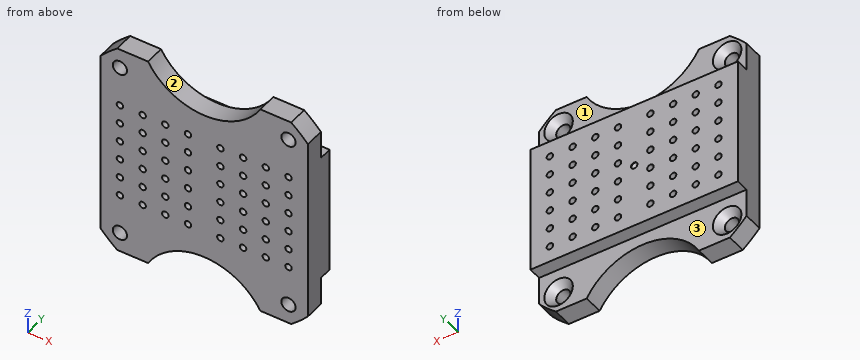
from build123d import *

# Parameters (mm, degrees)
SKIZZE1_W                                            = 32
SKIZZE1_H                                            = 33.6
AUFSATZ_LINEAR_AUSTRAGEN1_DEPTH                      = 5
SKIZZE9_R                                            = 0.5
SCHNITT_LINEAR_AUSTRAGEN1_DEPTH                      = 6
SKIZZE10_W                                           = 32
SKIZZE10_H                                           = 6.8
SCHNITT_LINEAR_AUSTRAGEN2_DEPTH                      = 2
FORMSENKUNG_F_R_M2_LINSENSENKSCHRAUBE_MI_D           = 2.2
FORMSENKUNG_F_R_M2_LINSENSENKSCHRAUBE_MI_DEPTH       = 4
FORMSENKUNG_F_R_M2_LINSENSENKSCHRAUBE_MI_CSINK_D     = 4.4
FORMSENKUNG_F_R_M2_LINSENSENKSCHRAUBE_MI_CSINK_ANGLE = 90
FORMSENKUNG_F_R_M2_LINSENSENKSCHRAUBE_MI_TIP         = 0.660946681
SKIZZE13_R                                           = 10
SCHNITT_LINEAR_AUSTRAGEN3_DEPTH                      = 24.393161394
SKIZZE14_R                                           = 31.5
SKIZZE14_R_2                                         = 21.5
SCHNITT_LINEAR_AUSTRAGEN_D_NN1_DEPTH                 = 10
F_1_0_1_DURCHMESSER_BOHRUNG1_D                       = 1
F_1_0_1_DURCHMESSER_BOHRUNG1_DEPTH                   = 0.1
F_1_0_1_DURCHMESSER_BOHRUNG1_TIP                     = 0.30043031


with BuildPart() as part:
    # Skizze1 → Aufsatz-Linear austragen1 (new body)
    with BuildSketch(Plane(origin=(0, 0, 0), x_dir=(1, 0, 0), z_dir=(0, 1, 0))):
        Rectangle(SKIZZE1_W, SKIZZE1_H)
    extrude(amount=AUFSATZ_LINEAR_AUSTRAGEN1_DEPTH)

    # Skizze9 → Schnitt-Linear austragen1 (cut)
    with BuildSketch(Plane(origin=(0, 5, 0), x_dir=(1, 0, 0), z_dir=(0, 1, 0))):
        with Locations(Location((-13, 7.5, 0), (0, 0, 270))):
            Circle(SKIZZE9_R)
        with Locations(Location((-9.5, 7.5, 0), (0, 0, 270))):
            Circle(SKIZZE9_R)
        with Locations(Location((-6, 7.5, 0), (0, 0, 270))):
            Circle(SKIZZE9_R)
        with Locations(Location((-2.5, 7.5, 0), (0, 0, 270))):
            Circle(SKIZZE9_R)
        with Locations(Location((-2.5, 4.5, 0), (0, 0, 270))):
            Circle(SKIZZE9_R)
        with Locations(Location((13, -7.5, 0), (0, 0, 270))):
            Circle(SKIZZE9_R)
        with Locations(Location((13, -4.5, 0), (0, 0, 270))):
            Circle(SKIZZE9_R)
        with Locations(Location((13, -1.5, 0), (0, 0, 270))):
            Circle(SKIZZE9_R)
        with Locations(Location((13, 1.5, 0), (0, 0, 270))):
            Circle(SKIZZE9_R)
        with Locations(Location((13, 4.5, 0), (0, 0, 270))):
            Circle(SKIZZE9_R)
        with Locations(Location((-2.5, 1.5, 0), (0, 0, 270))):
            Circle(SKIZZE9_R)
        with Locations(Location((-9.5, 4.5, 0), (0, 0, 270))):
            Circle(SKIZZE9_R)
        with Locations(Location((-6, 4.5, 0), (0, 0, 270))):
            Circle(SKIZZE9_R)
        with Locations(Location((-2.5, -1.5, 0), (0, 0, 270))):
            Circle(SKIZZE9_R)
        with Locations(Location((-2.5, -4.5, 0), (0, 0, 270))):
            Circle(SKIZZE9_R)
        with Locations(Location((-2.5, -7.5, 0), (0, 0, 270))):
            Circle(SKIZZE9_R)
        with Locations(Location((6, -7.5, 0), (0, 0, 270))):
            Circle(SKIZZE9_R)
        with Locations(Location((9.5, -7.5, 0), (0, 0, 270))):
            Circle(SKIZZE9_R)
        with Locations(Location((2.5, -7.5, 0), (0, 0, 270))):
            Circle(SKIZZE9_R)
        with Locations(Location((2.5, -4.5, 0), (0, 0, 270))):
            Circle(SKIZZE9_R)
        with Locations(Location((6, -4.5, 0), (0, 0, 270))):
            Circle(SKIZZE9_R)
        with Locations(Location((-9.5, 1.5, 0), (0, 0, 270))):
            Circle(SKIZZE9_R)
        with Locations(Location((-6, 1.5, 0), (0, 0, 270))):
            Circle(SKIZZE9_R)
        with Locations(Location((2.5, -1.5, 0), (0, 0, 270))):
            Circle(SKIZZE9_R)
        with Locations(Location((2.5, 1.5, 0), (0, 0, 270))):
            Circle(SKIZZE9_R)
        with Locations(Location((9.5, -4.5, 0), (0, 0, 270))):
            Circle(SKIZZE9_R)
        with Locations(Location((2.5, 4.5, 0), (0, 0, 270))):
            Circle(SKIZZE9_R)
        with Locations(Location((2.5, 7.5, 0), (0, 0, 270))):
            Circle(SKIZZE9_R)
        with Locations(Location((6, -1.5, 0), (0, 0, 270))):
            Circle(SKIZZE9_R)
        with Locations(Location((9.5, -1.5, 0), (0, 0, 270))):
            Circle(SKIZZE9_R)
        with Locations(Location((-9.5, -1.5, 0), (0, 0, 270))):
            Circle(SKIZZE9_R)
        with Locations(Location((-6, -1.5, 0), (0, 0, 270))):
            Circle(SKIZZE9_R)
        with Locations(Location((6, 1.5, 0), (0, 0, 270))):
            Circle(SKIZZE9_R)
        with Locations(Location((9.5, 1.5, 0), (0, 0, 270))):
            Circle(SKIZZE9_R)
        with Locations(Location((6, 4.5, 0), (0, 0, 270))):
            Circle(SKIZZE9_R)
        with Locations(Location((-9.5, -4.5, 0), (0, 0, 270))):
            Circle(SKIZZE9_R)
        with Locations(Location((-6, -4.5, 0), (0, 0, 270))):
            Circle(SKIZZE9_R)
        with Locations(Location((9.5, 4.5, 0), (0, 0, 270))):
            Circle(SKIZZE9_R)
        with Locations(Location((6, 7.5, 0), (0, 0, 270))):
            Circle(SKIZZE9_R)
        with Locations(Location((9.5, 7.5, 0), (0, 0, 270))):
            Circle(SKIZZE9_R)
        with Locations(Location((13, 7.5, 0), (0, 0, 270))):
            Circle(SKIZZE9_R)
        with Locations(Location((-9.5, -7.5, 0), (0, 0, 270))):
            Circle(SKIZZE9_R)
        with Locations(Location((-6, -7.5, 0), (0, 0, 270))):
            Circle(SKIZZE9_R)
        with Locations(Location((-13, 4.5, 0), (0, 0, 270))):
            Circle(SKIZZE9_R)
        with Locations(Location((-13, 1.5, 0), (0, 0, 270))):
            Circle(SKIZZE9_R)
        with Locations(Location((-13, -1.5, 0), (0, 0, 270))):
            Circle(SKIZZE9_R)
        with Locations(Location((-13, -4.5, 0), (0, 0, 270))):
            Circle(SKIZZE9_R)
        with Locations(Location((-13, -7.5, 0), (0, 0, 270))):
            Circle(SKIZZE9_R)
    extrude(amount=-SCHNITT_LINEAR_AUSTRAGEN1_DEPTH, mode=Mode.SUBTRACT)

    # Skizze10 → Schnitt-Linear austragen2 (cut)
    with BuildSketch(Plane(origin=(0, 5, 0), x_dir=(1, 0, 0), z_dir=(0, 1, 0))):
        with Locations((0, 13.4)):
            Rectangle(SKIZZE10_W, SKIZZE10_H)
        with Locations((0, -13.4)):
            Rectangle(SKIZZE10_W, SKIZZE10_H)
    extrude(amount=-SCHNITT_LINEAR_AUSTRAGEN2_DEPTH, mode=Mode.SUBTRACT)

    # Formsenkung für M2 Linsensenkschraube mit Schlitz2
    with Locations(Plane(origin=(0, 3, 0), x_dir=(1, 0, 0), z_dir=(0, 1, 0))):
        with Locations((-13, 13.75), (13, 13.75), (13, -13.75), (-13, -13.75)):
            CounterSinkHole(FORMSENKUNG_F_R_M2_LINSENSENKSCHRAUBE_MI_D / 2, FORMSENKUNG_F_R_M2_LINSENSENKSCHRAUBE_MI_CSINK_D / 2, depth=FORMSENKUNG_F_R_M2_LINSENSENKSCHRAUBE_MI_DEPTH, counter_sink_angle=FORMSENKUNG_F_R_M2_LINSENSENKSCHRAUBE_MI_CSINK_ANGLE)
            with Locations((0, 0, -(FORMSENKUNG_F_R_M2_LINSENSENKSCHRAUBE_MI_DEPTH + FORMSENKUNG_F_R_M2_LINSENSENKSCHRAUBE_MI_TIP / 2))):  # 118° drill point
                Cone(0, FORMSENKUNG_F_R_M2_LINSENSENKSCHRAUBE_MI_D / 2, FORMSENKUNG_F_R_M2_LINSENSENKSCHRAUBE_MI_TIP, mode=Mode.SUBTRACT)

    # Skizze13 → Schnitt-Linear austragen3 (cut, through all)
    with BuildSketch(Plane(origin=(0, 3, 0), x_dir=(1, 0, 0), z_dir=(0, 1, 0))):
        with Locations((0, 21.8)):
            Circle(SKIZZE13_R)
    schnitt_linear_austragen3 = extrude(amount=-SCHNITT_LINEAR_AUSTRAGEN3_DEPTH, mode=Mode.SUBTRACT)

    # Spiegeln3: Schnitt-Linear austragen3 across plane
    add(schnitt_linear_austragen3.mirror(Plane.XY), mode=Mode.SUBTRACT)

    # Skizze14 → Schnitt-Linear-Austragen-Dünn1 (cut)
    with BuildSketch(Plane(origin=(0, 5, 0), x_dir=(1, 0, 0), z_dir=(0, 1, 0))):
        Circle(SKIZZE14_R)
        Circle(SKIZZE14_R_2, mode=Mode.SUBTRACT)
    extrude(amount=-SCHNITT_LINEAR_AUSTRAGEN_D_NN1_DEPTH, mode=Mode.SUBTRACT)

    # Ø1.0 (1) Durchmesser Bohrung1
    with Locations(Plane(origin=(0, 5, 0), x_dir=(1, 0, 0), z_dir=(0, 1, 0))):
        with Locations((0, 0)):
            Hole(F_1_0_1_DURCHMESSER_BOHRUNG1_D / 2, depth=F_1_0_1_DURCHMESSER_BOHRUNG1_DEPTH)
            with Locations((0, 0, -(F_1_0_1_DURCHMESSER_BOHRUNG1_DEPTH + F_1_0_1_DURCHMESSER_BOHRUNG1_TIP / 2))):  # 118° drill point
                Cone(0, F_1_0_1_DURCHMESSER_BOHRUNG1_D / 2, F_1_0_1_DURCHMESSER_BOHRUNG1_TIP, mode=Mode.SUBTRACT)


solid = part.part
The listing builds one solid part. Answer for the finished solid, in the listing's coordinates (mm). Face numbers are marked on the shaded views. A direction names the side the tool comes from. Coordinates: 2 decimals unless noted, no trailing zeros. Order: outer loops, then holes, each group sorted by start corner. A loop starts at its lowest first (then second) coordinate and runs counter-clockwise, first axis right, second up. Notation, with made-up numbers: M -29,65 L -19,65 A13 ccw -19,75 Z; hole C -9,86 d1. An arc over 180 degrees is marked long. Use CSV: the item, a comma, the result in double quotes.
Q1. Given pin 1 Ø1.8 at (x, z) = (13, -13.75) entering from -Y; pin 2 Ø4 at (x, z) = (-3, 13.5) entering from +Y; pin 3 Ø1.6 at (x, y) = (3.5, 3.5) entering from -Z; pin 4 Ø1 at (x, y) = (1.5, 4) entering from +Z, each flat-ended and moving along its own axis, determine where each tip first touches the part or whether it passes through.
Here are the results:
pin 1,"through"
pin 2,"y = 3"
pin 3,"z = -12.69"
pin 4,"z = 10"
Q2. Section A-A (z = -13.75) is taken. Determine the outline of the cut face in (x, y), then the cut area to 3 significant figures.
Here are the results:
outline,"M -16,0 L -14.1,0 L -14.1,1.9 L -15.2,3 L -16,3 Z; M -11.9,0 L -5.93,0 L -5.93,3 L -10.8,3 L -11.9,1.9 Z; M 5.93,0 L 11.9,0 L 11.9,1.9 L 10.8,3 L 5.93,3 Z; M 14.1,0 L 16,0 L 16,3 L 15.2,3 L 14.1,1.9 Z"
area,"44.8 mm2"
Q3. Straight lines are drawn through the part: L1, parallel to X at y = 2.2, z = 13; L2, parallel to Z at x = 8, y = 3.4; L3, parallel to Y at x = 9, z = -12.5. For each, find the intervals that lie inside material, in ascending order.
Here are the results:
L1,"-16 to -14.18, -11.82 to -4.75, 4.75 to 11.82, 14.18 to 16"
L2,"-10 to 10"
L3,"0 to 3"
Q4. A tool of negligible diameter and unlimited length cuts with its end or side. For the marked faces 1, 2 and 3, from which of +Z, -Z, +X, -X, +Y, -Y can it reach the whole face along a straight path? Write none if from no direction.
Here are the results:
face 1,"+Z, +X, -X, +Y"
face 2,"+Z, +Y, -Y"
face 3,"-Z, +X, -X, +Y"
Q5. Section D-D (x = 4) is taken. Determine the outline of the cut face in (y, z), then the cut area to 3 significant figures.
Here are the results:
outline,"M 0,-12.63 L 3,-12.63 L 3,-10 L 5,-10 L 5,10 L 3,10 L 3,12.63 L 0,12.63 Z"
area,"116 mm2"
Q6. Section B-B (z = 7.5) is taken. Give the number of separate pieces and of enclosed holes in the cut face, then the cut area to 3 significant figures.
Here are the results:
separate pieces,"9"
enclosed holes,"0"
area,"120 mm2"
